Geometry: final body of the model. Coordinates: model frame, mm. A direction names the side the tool comes from. Round coordinates to 2 decimals unless told otherwise and drop trailing zeros. Loops run counter-clockwise (first coordinate to the right, second up) from the corner with the lowest first, then second, coordinate; pieces in that order, holes last. Notation, with made-up numbers: (62.25, -33.75) -> (114.25, -33.75) arc R18 cw to (114.25, -16.75) -> close; hole circle Ø3 at (4.5, 74). An arc over 180 degrees is marked (long way). Answer in a Markdown table with one row per item.
```python
from build123d import *

# Parameters (mm, degrees)
F1_ANGLE = 10
F2_R     = 5
F3_R     = 1


# Not quite as in the source:
# - a feature names something its author has since deleted; it is built from what else it names


with BuildPart() as f1:
    # F0 (on Front) → F1 (revolve)
    with BuildSketch(Plane.XZ):
        Polygon((-3, 0), (0, 0), (0, 15.8), (2.9, 15.8), (2.9, 6.3), (1.4, 6.3), (1.4, 1.8), (5.9, 1.8), (5.9, 18.8), (0.0073256942, 18.8), (-3, 18.8), align=None)
        Polygon((-0.552561582, 53.8), (-3, 18.8), (0.0073256942, 18.8), (2.4547641123, 53.8), align=None)
        Polygon((-0.552561582, 76.1240777928), (-0.552561582, 53.8), (2.4547641123, 53.8), (12.7011916374, 53.8), (12.7011916374, 56.8), (2.7011916374, 57.3240777928), (2.7011916374, 76.1240777928), align=None)
    revolve(axis=Axis((56.5, 0, 26.2500001118), (0, 0, -1)), revolution_arc=F1_ANGLE)

    # F2
    f2_edges = [f1.edges().sort_by_distance(p)[0] for p in [
        (0.222297, 4.923661, 18.8),
        (2.660423, 4.710353, 53.8),
    ]]
    fillet(f2_edges, radius=F2_R)

    # F3
    f3_edges = [f1.edges().sort_by_distance(p)[0] for p in [
        (6.092548, 4.410081, 1.8),
        (6.092548, 4.410081, 18.8),
        (12.867859, 3.817318, 53.8),
        (2.905912, 4.688875, 76.124078),
        (-0.335459, 4.972458, 76.124078),
    ]]
    fillet(f3_edges, radius=F3_R)


solid = f1.part
```
Item 1: Cut plane A-A (z = 63). Output: boundary loops of the cut face in (x, y).
Answer:
| item | result |
|---|---|
| outline | (-0.55, 0) -> (2.7, 0) arc R53.8 cw to (3.52, 9.34) -> (0.31, 9.91) arc R57.05 ccw to start |
Item 2: Pin query (flat end, axial travel): pin 1 Ø2 at (x, z) = (3.5, 22.5) entering from +Y; pin 2 Ø3 at (y, z) = (2, 24.5) entering from -X; pin 3 Ø5 at (y, z) = (5, 65) entering from +X; pin 4 Ø1.3 at (x, y) = (3, 3.5) entering from -Z. Return the tip coordinate at first contact, or that it passes through.
Answer:
| item | result |
|---|---|
| pin 1 | passes through |
| pin 2 | stops at x = -2.68 |
| pin 3 | stops at x = 3.23 |
| pin 4 | stops at z = 1.8 |
Item 3: Cut plane B-B (z = 51). Output: boundary loops of the cut face in (x, y), then the cut area to 3 significant figures.
Answer:
| item | result |
|---|---|
| outline | (-0.75, 0) -> (2.63, 0) arc R53.87 cw to (3.45, 9.35) -> (0.12, 9.94) arc R57.25 ccw to start |
| area | 32.7 mm² |
Item 4: Draft query along X for faces 6 (the face through (4, 5, 1.8)), 7 (the face through (1.472, 4.747, 36.824)), 8 (the face through (0.21, 4.86, 8.01)). Return one class per face: pulls with the +X half, pulls with the -X half, needs draft (parallel to the pull), parting line crosses it, or undercut.
Answer:
| item | result |
|---|---|
| face 6 | needs draft |
| face 7 | pulls with the +X half |
| face 8 | undercut |
Item 5: Line query: probe 1 along X at (y, z) = (2.75, 8); probe 2 along X at (y, z) = (0.5, 13); probe 3 along X at (y, z) = (1, 62.5). Output: solid intervals per line, ascending. Write a range as [from, to].
Answer:
| item | result |
|---|---|
| probe 1 | x = [-2.94, 0.07], [2.97, 5.97] |
| probe 2 | x = [-3, 0], [2.9, 5.9] |
| probe 3 | x = [-0.54, 2.71] |
Item 6: Reachability of faces 1 (the face through (-0.34, 4.9, 64.31)), 2 (the face through (12.863, 3.764, 55.814)), 3 (the face through (2.9, 4.6, 66.3)), 4 (the face through (1.6, 4.7, 4)), 5 (the face through (2.5, 4.9, 6.3)) from +Z, -Z, +X, -X, +Y, -Y: full face, straight path, thin tool, end or side. Return the list, or none.
Answer:
| item | result |
|---|---|
| face 1 | +Z, -X, +Y |
| face 2 | +Z, -Z, +X, -Y |
| face 3 | +Z, +X, -Y |
| face 4 | -Z, +Y |
| face 5 | +Y |
